Autodesk Inventor part; units mm, degrees
ref_plane "YZ Plane" through (0, 0, 0) normal (1, 0, 0) x (0, 1, 0)
ref_plane "XZ Plane" through (0, 0, 0) normal (0, 1, 0) x (-1, 0, 0)
ref_plane "XY Plane" through (0, 0, 0) normal (0, 0, 1) x (1, 0, 0)
sketch "Sketch1" plane through (0, 0, 0) normal (1, 0, 0) x (0, 1, 0)
  circle A0 centre (0, 0) radius 4.7625
  circle A1 centre (0, 0) radius 19.05
  dimension "d0" = 9.525
  dimension "d1" = 38.1
extrude "Extrusion1" add sketch "Sketch1" along normal blind 12.7
sketch "Sketch2" plane through (12.7, 0, 0) normal (1, 0, 0) x (0, 0, -1)
  circle A0 centre (0, 0) radius 19.05
  line L0 (0, -19.05) -> (-50.8, -19.05)
  circle A1 centre (0, 0) radius 4.7625
  line L1 (0, -19.05) -> (11.4002, -19.05)
  line L2 (-13.4704, 13.4704) -> (-25.8301, 1.1106)
  line L3 (0, 0) -> (-13.4704, 13.4704)
  line L4 (0, 0) -> (-19.05, 0)
  line L5 (-25.8301, 1.1106) -> (-26.9408, 0)
  line L6 (0, -19.05) -> (-127, -19.05)
  line L7 (0, -38.1) -> (0, -19.05)
  line L8 (-26.9408, 0) -> (-59.9363, -19.05)
  line L9 (0, -28.575) -> (-127, -28.575)
  line L10 (-127, -28.575) -> (-100.8303, -19.05)
  line L11 (-79.2802, -19.05) -> (16.9609, 15.9789)
  dimension "d6" = 50.8
  dimension "d7" = 0
  dimension "d8" = 180
  dimension "d9" = 45
  dimension "d10" = 45
  dimension "d11" = 17.4793
  dimension "d13" = 19.05
  dimension "d17" = 30
  dimension "d18" = 180
  dimension "d19" = 38.1
  dimension "d20" = 127
  dimension "d21" = 20
  dimension "d24" = 20
  dimension "d25" = 0
extrude "Extrusion2" add sketch "Sketch2" against normal blind 12.7 contours A0 L0 L6 L8 L11 | L7 L9 L10 L6 L0 | L11 L5 L2 A0
sketch "Sketch3" plane through (12.7, 0, 0) normal (1, 0, 0) x (0, 0, -1)
  line L0 (-59.9363, -19.05) -> (-26.9408, 0)
  line L1 (-26.9408, 0) -> (-79.2802, -19.05)
  line L2 (-100.8303, -19.05) -> (-59.9363, -19.05)
  line L3 (-79.2802, -19.05) -> (-59.9363, -19.05)
  line L4 (-26.9408, 0) -> (-59.9363, -19.05)
  point P0 (0, 0)
  dimension "d26" = 20
extrude "Extrusion3" add sketch "Sketch3" against normal blind 12.7
fillet "Fillet1" radius 9.525 1 edges at (6.35, -28.575, 0)
fillet "Fillet2" radius 9.525 2 edges at (6.35, -19.0505, 0) (6.35, -19.05, 0)
sketch "Sketch4" plane through (12.7, 0, 0) normal (1, 0, 0) x (0, 0, -1)
  point P0 (0, 0)
properties part number "Wedgelet" material "Steel"
Can you work these out from the model? Positions are in its coordinate system, mm. A direction names the side the tool comes from. Round coordinates to 2 decimals unless told otherwise and drop trailing zeros. Write each loop counter-clockwise with the first axis right and the second up, starting at its lowest first coordinate (ties: lowest second). Pieces come first, ordered by that corner, then holes. Notation, with made-up numbers: (-4.75, -24) -> (50.25, -24) arc R22 cw to (50.25, -10) -> close; hole circle Ø8 at (35, -34). An arc over 180 degrees is marked (long way). Use one line per item in the form item = value. Start each with the question number.
Q1. Imagine slicing it at B-B (z = 86.5). Please give me the cut outline in (x, y) (3 decimals).
Q2. Imagine slicing it at C-C (y = -17). Please give me the cut outline in (x, z).
Q3. Which directions (+Z, -Z, +X, -X, +Y, -Y) give clear straight access to the entire face, cutting with the end or side of a thin tool? Please do faces 1 (the face through (0, -10, 23)), 2 (the face through (6, -19.05, 90)).
Q4. If I drill on probe 1 along Z at (x, y) = (11.25, 3); probe 2 along Y at (x, z) = (8, 75) (3 decimals); probe 3 along Z at (x, y) = (6.75, 5), over which ranges is the centre line in solid material (lowest first)? Write a range as [from, to].
Q5. I'm going to push flat-ended pins straight in: P1, Ø3, axis at x = 11, y = 7, coming from the +Z side; P2, Ø5, axis at x = 2.5, z = 44, coming from the +Y side; P3, Ø5.5, axis at y = 0, z = 0, coming from the +X side. Where does each tip first touch, or does it pass through?
Q6. Imagine slicing it at A-A (y = 3.5). Please give me the cut outline in (x, z).
Q7. We'd pull the mould along Z, two halves only. Please class faces 3 (the face through (6.44, -23.88, 114.1)), 4 (the face through (6.26, -3.78, 2.9)), 5 (the face through (12.7, -10, 23)): +Z half, -Z half, draft (parallel to the pull), parting line (faces both ways), or undercut.
Worked out:
q1.outline = (0, -28.575) -> (12.7, -28.575) -> (12.7, -19.05) -> (0, -19.05) -> close
q2.outline = (0, -8.6) -> (12.7, -8.6) -> (12.7, 73.65) -> (0, 73.65) -> close
q3.face_1 = +Z, -Z, -X, +Y, -Y
q3.face_2 = +Z, +X, -X, +Y
q4.probe_1 = [-18.81, -3.7], [3.7, 23.94]
q4.probe_2 = [-28.575, -17.492]
q4.probe_3 = [-18.38, 21.94]
q5.P1 = 21.44
q5.P2 = -5.3
q5.P3 = through
q6.outline = (0, -18.73) -> (12.7, -18.73) -> (12.7, -3.23) -> (0, -3.23) -> close; (0, 3.23) -> (12.7, 3.23) -> (12.7, 23.44) -> (0, 23.44) -> close
q7.face_3 = +Z half
q7.face_4 = undercut
q7.face_5 = draft
